The model under review builds one solid part; all positions refer to its coordinate system, in mm. Face numbers are marked on the shaded views. A direction names the side the tool comes from. Give positions to 0.01 mm unless a question says otherwise; leave off trailing zeros. Order: outer loops, then holes, each group sorted by start corner. A loop starts at its lowest first (then second) coordinate and runs counter-clockwise, first axis right, second up. Notation, with made-up numbers: M 33.5,73.5 L 67.5,73.5 A17 ccw 67.5,80.5 Z; hole C 64,16 d4. An arc over 180 degrees is marked long. One line per question, with ' | ' between items. Start each with the question number.
1. We need section A-A on z = 24.25. Write out the cut boundary in (x, y).
2. Wall thickness on L1, parallel to Z at x = 14.5, y = 7; L2, parallel to Z at x = 15, y = 8; L3, parallel to X at y = 3.5, z = 9.75: over which ranges is each line inside the solid? List them lowest first.
3. The part is to be moulded in two halves that separate along Z. For the marked faces 3, 4 and 5, say which applies: +Z half, -Z half, draft (parallel to the pull), parting line (faces both ways), or undercut.
4. We need section B-B on y = 9. Count the separate pieces of the cut face and the enclosed holes in it, then the cut area to 3 significant figures.
5. Insertion check: P1, Ø1.5, axis at x = 8.5, z = 16.5, coming from the +Y side; P2, Ø4, axis at x = 21, y = 17.5, coming from the -Z side; P3, Ø6, axis at x = 7, z = 11.5, coming from the +Y side. Each pin has a flat end and moves straight along its axis. Give the tip position at first contact, or say it passes through.
6. For the marked faces 1 and 2, list the 3-axis set-ups (+Z, -Z, +X, -X, +Y, -Y) from which the entire face can be reached by the end or side of a thin tool; tool diameter is ignored.
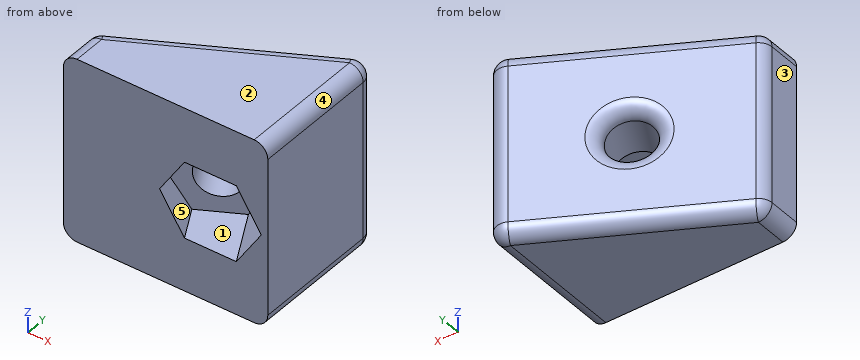
```python
from build123d import *

# Parameters (mm, degrees)
SKETCH1_W           = 30
SKETCH1_H           = 27
BOSS_EXTRUDE1_DEPTH = 22
CUT_EXTRUDE1_DEPTH  = 46.967379738
CUT_EXTRUDE2_DEPTH  = 46.66149711
SKETCH4_R           = 6.960577045
SKETCH4_R_2         = 3.3
BOSS_EXTRUDE2_DEPTH = 8
FILLET2_R           = 2


with BuildPart() as part:
    # Sketch1 → Boss-Extrude1 (new body)
    with BuildSketch(Plane(origin=(0, 0, 0), x_dir=(1, 0, 0), z_dir=(0, 1, 0))):
        with Locations((15, -13.5)):
            Rectangle(SKETCH1_W, SKETCH1_H)
    extrude(amount=BOSS_EXTRUDE1_DEPTH)

    # Sketch2 → Cut-Extrude1 (cut, through all)
    with BuildSketch(Plane.XY.offset(27)):
        Polygon((0, 6), (0, 22), (30, 22), align=None)
    extrude(amount=-CUT_EXTRUDE1_DEPTH, mode=Mode.SUBTRACT)

    # Sketch3 → Cut-Extrude2 (cut, through all)
    with BuildSketch(Plane(origin=(-2.491349481, 4.671280277, 0), x_dir=(0.8823529411764706, 0.47058823529411764, 0), z_dir=(-0.47058823529411764, 0.8823529411764706, 0))):
        Polygon((22.394089302, -19.014916182), (25.627250808, -13.414916183), (22.394089302, -7.814916185), (19.036531329, -7.814916185), (15.678973356, -7.814916185), (12.445811849, -13.414916183), (15.678973356, -19.014916182), (19.036531329, -19.014916182), align=None)
    extrude(amount=-CUT_EXTRUDE2_DEPTH, mode=Mode.SUBTRACT)

    # Sketch4 → Boss-Extrude2 (add)
    with BuildSketch(Plane(origin=(-2.491349481, 4.671280277, 0), x_dir=(0.8823529411764706, 0.47058823529411764, 0), z_dir=(-0.47058823529411764, 0.8823529411764706, 0))):
        with Locations((19.036531329, -13.414916183)):
            Circle(SKETCH4_R)
        with Locations(Location((19.036531329, -13.414916183, 0), (0, 0, 180))):
            Circle(SKETCH4_R_2, mode=Mode.SUBTRACT)
    extrude(amount=-BOSS_EXTRUDE2_DEPTH)

    # Fillet2
    fillet2_edges = [part.edges().sort_by_distance(p)[0] for p in [
        (30, 22, 13.5),
        (0, 3, 0),
        (0, 3, 27),
        (15, 14, 0),
        (0, 6, 13.5),
        (15, 14, 27),
        (17.217354633, 15.182589137, 13.414916183),
        (30, 11, 0),
        (30, 11, 27),
    ]]
    fillet(fillet2_edges, radius=FILLET2_R)


solid = part.part
```
Entries:
1) outline: M 0,0 L 30,0 L 30,18.67 A2 ccw 27.06,20.43 L 1.06,6.56 A2 ccw 0,4.8 Z
2) L1: z = 0 to 11.93, 14.9 to 27 | L2: z = 0 to 10.82, 16.01 to 27 | L3: x = 0 to 14.64, 24.78 to 30
3) face 3: draft | face 4: +Z half | face 5: undercut
4) separate pieces: 1 | enclosed holes: 2 | area: 610 mm^2
5) P1: stops at y = 10.93 | P2: stops at z = 0.02 | P3: stops at y = 11.33
6) face 1: none | face 2: +Z, +X, -X, +Y, -Y
